Here's how the part is built. I have some questions about the finished solid (model axes, mm). A direction names the side the tool comes from. Coordinates: 2 decimals unless noted, no trailing zeros. Write each loop counter-clockwise with the first axis right and the second up, starting at its lowest first coordinate (ties: lowest second). Pieces come first, ordered by that corner, then holes. Notation, with made-up numbers: (52.25, -19.5) - (108.25, -19.5) arc R15 ccw to (108.25, 3.5) - close; hole circle Ø3 at (28.5, -10). An arc over 180 degrees is marked (long way). Answer in a Markdown table with one row per item. Add a question column.
Item 1: Which directions (+Z, -Z, +X, -X, +Y, -Y) give clear straight access to the entire face, cutting with the end or side of a thin tool? Please do faces 1 (the face through (74, 0, 1)), 2 (the face through (131, 18, 1)), 3 (the face through (129.633, 4, 1)), 4 (the face through (-8.367, 21, 1)).
Item 2: Imagine slicing it at A-A (x = 26). Please give me the cut outline in (y, z).
Item 3: If I drill on probe 1 along X at (y, z) = (36, 0.5); probe 2 along Y at (x, z) = (0.5, 0.45); probe 3 along X at (y, z) = (6, 2), over which ranges is the centre line in solid material (lowest first)? Write a range as from..to.
Item 4: Imagine slicing it at B-B (y = 24.5). Please give me the cut outline in (x, z), plus the area to 3 significant figures.
Item 5: We'd pull the mould along X, two halves only. Please class faces 5 (the face through (-2.367, 34, 1)), 6 (the face through (54.633, -1, 1)), 7 (the face through (122.633, 33, 1)), 8 (the face through (125, 0, 1)): +X half, -X half, draft (parallel to the pull), parting line (faces both ways), or undercut.
Item 6: I'm going to push flat-ended pins straight in: pin 1 (1.5 mm diameter, centred on y = -1.5, z = 2, fed in from -X); pin 2 (0.9 mm diameter, centred on y = 31, z = 1, fed in from -X); pin 3 (1.5 mm diameter, centred on x = -2, z = 1.5, fed in from -Y). Where does each tip first touch, or does it pass through?
from build123d import *

# Parameters (mm, degrees)
BOSS_EXTRUDE1_DEPTH = 3


with BuildPart() as part:
    # Sketch1 → Boss-Extrude1 (new body)
    with BuildSketch(Plane.XY):
        Polygon((14.633144841, 0), (27.633144841, 0), (27.633144841, -3), (40.633144841, -3), (40.633144841, 0), (54.633144841, 0), (54.633144841, -3), (67.633144841, -3), (67.633144841, 0), (80.633144841, 0), (80.633144841, -3), (93.633144841, -3), (93.633144841, 0), (106.633144841, 0), (106.633144841, -3), (119.633144841, -3), (119.633144841, 0), (125, 0), (129.633144841, 0), (129.633144841, 8), (132.633144841, 8), (132.633144841, 18), (129.633144841, 18), (129.633144841, 23), (122.633144841, 23), (122.633144841, 44), (-2.366855159, 44), (-2.366855159, 23), (-8.366855159, 23), (-8.366855159, 18), (-11.366855159, 18), (-11.366855159, 8), (-8.366855159, 8), (-8.366855159, 0), (0, 0), (1.633144841, 0), (1.633144841, -3), (14.633144841, -3), align=None)
    extrude(amount=BOSS_EXTRUDE1_DEPTH)


solid = part.part
Here are the results:
| question | item | result |
|---|---|---|
| 1 | face 1 | +Z, -Z, -Y |
| 1 | face 2 | +Z, -Z, +X, +Y |
| 1 | face 3 | +Z, -Z, +X, -Y |
| 1 | face 4 | +Z, -Z, -X, +Y |
| 2 | outline | (0, 0) - (44, 0) - (44, 3) - (0, 3) - close |
| 3 | probe 1 | x = -2.37..122.63 |
| 3 | probe 2 | y = 0..44 |
| 3 | probe 3 | x = -8.37..129.63 |
| 4 | outline | (-2.37, 0) - (122.63, 0) - (122.63, 3) - (-2.37, 3) - close |
| 4 | area | 375 mm2 |
| 5 | face 5 | -X half |
| 5 | face 6 | undercut |
| 5 | face 7 | +X half |
| 5 | face 8 | draft |
| 6 | pin 1 | stops at x = 1.63 |
| 6 | pin 2 | stops at x = -2.37 |
| 6 | pin 3 | stops at y = 0 |
